Read the model definition and answer for the solid it produces. Units are mm, in the model's axes. Give positions to 0.01 mm unless a question says otherwise; leave off trailing zeros. Loops run counter-clockwise (first coordinate to the right, second up) from the corner with the lowest first, then second, coordinate; pieces in that order, holes last. Notation, with made-up numbers: (47, -30.75) -> (97, -30.75) arc R21 ccw to (97, 0.25) -> close; hole circle Ø1 at (-40, -27). An arc over 180 degrees is marked (long way). Return JSON: item names as keys, results as strings. Group by question number.
from build123d import *

# Parameters (mm, degrees)
SKETCH_1_R               = 35.5
EXTRUDE_1_DEPTH          = 3
CUT_EXTRUDE_1_REACH      = 193.4
SKETCH_3_R               = 2
PATTERN_CIRCULAR_1_COUNT = 10
MIRROR_1_COPY_1_REACH    = 193.4
MIRROR_1_COPY_1_SKETCH_R = 2
MIRROR_1_COPY_2_REACH    = 193.4
MIRROR_1_COPY_2_SKETCH_R = 2
MIRROR_1_COPY_3_REACH    = 193.4
MIRROR_1_COPY_3_SKETCH_R = 2
MIRROR_1_COPY_4_REACH    = 193.4
MIRROR_1_COPY_4_SKETCH_R = 2
MIRROR_1_COPY_5_REACH    = 193.4
MIRROR_1_COPY_5_SKETCH_R = 2
MIRROR_1_COPY_6_REACH    = 193.4
MIRROR_1_COPY_6_SKETCH_R = 2
MIRROR_1_COPY_7_REACH    = 193.4
MIRROR_1_COPY_7_SKETCH_R = 2
MIRROR_1_COPY_8_REACH    = 193.4
MIRROR_1_COPY_8_SKETCH_R = 2
MIRROR_1_COPY_9_REACH    = 193.4
MIRROR_1_COPY_9_SKETCH_R = 2
CUT_EXTRUDE_2_REACH      = 193.4
SKETCH_4_R               = 1.5
PATTERN_LINEAR_1_COUNT   = 5
PATTERN_LINEAR_1_PITCH   = 21
CUT_EXTRUDE_3_REACH      = 193.4
SKETCH_6_R               = 1.5
PATTERN_LINEAR_3_COUNT   = 5
PATTERN_LINEAR_3_PITCH   = 15
MIRROR_2_COPY_1_REACH    = 193.4
MIRROR_2_COPY_1_SKETCH_R = 1.5
MIRROR_2_COPY_2_REACH    = 193.4
MIRROR_2_COPY_2_SKETCH_R = 1.5
MIRROR_2_COPY_3_REACH    = 193.4
MIRROR_2_COPY_3_SKETCH_R = 1.5
MIRROR_2_COPY_4_REACH    = 193.4
MIRROR_2_COPY_4_SKETCH_R = 1.5
CUT_EXTRUDE_4_REACH      = 193.4
SKETCH_7_R               = 1.5
PATTERN_LINEAR_4_COUNT   = 2
PATTERN_LINEAR_4_PITCH   = 50


with BuildPart() as part:
    # Sketch 1 → Extrude 1 (new body)
    with BuildSketch(Plane(origin=(0, 0, 0), x_dir=(1, 0, 0), z_dir=(0, 1, 0))):
        with BuildLine():
            Line((-150, 65), (150, 65))
            ThreePointArc((150, 65), (171.213203436, 56.213203436), (180, 35))
            Line((180, 35), (180, -35))
            ThreePointArc((180, -35), (171.213203436, -56.213203436), (150, -65))
            Line((150, -65), (-150, -65))
            ThreePointArc((-150, -65), (-171.213203436, -56.213203436), (-180, -35))
            Line((-180, -35), (-180, 35))
            ThreePointArc((-180, 35), (-171.213203436, 56.213203436), (-150, 65))
        make_face()
        with Locations(Location((105, 0, 0), (0, 0, 270))):
            Circle(SKETCH_1_R, mode=Mode.SUBTRACT)
        with Locations(Location((-105, 0, 0), (0, 0, 270))):
            Circle(SKETCH_1_R, mode=Mode.SUBTRACT)
    extrude(amount=EXTRUDE_1_DEPTH)

    # Sketch 3 → Cut-Extrude 1 (cut, up to next)
    with BuildSketch(Plane(origin=(0, 3, 0), x_dir=(1, 0, 0), z_dir=(0, 1, 0)), mode=Mode.PRIVATE) as cut_extrude_1_sk1:
        with Locations(Location((-63, 0, 0), (0, 0, 270))):
            Circle(SKETCH_3_R)
    cut_extrude_1_tool1 = extrude(cut_extrude_1_sk1.sketch, amount=-CUT_EXTRUDE_1_REACH, mode=Mode.PRIVATE) & part.part
    cut_extrude_1 = cut_extrude_1_tool1.solids().sort_by_distance((-63, 3, 0))[0]
    add(cut_extrude_1, mode=Mode.SUBTRACT)

    # Pattern Circular 1: Cut-Extrude 1 ×10 about axis
    pattern_circular_1_axis = Axis((-105, 0, 0), (0, 1, 0))
    for i in range(1, PATTERN_CIRCULAR_1_COUNT):
        add(cut_extrude_1.rotate(pattern_circular_1_axis, i * 360 / PATTERN_CIRCULAR_1_COUNT), mode=Mode.SUBTRACT)

    # Mirror 1: Cut-Extrude 1 across plane
    add(cut_extrude_1.mirror(Plane(origin=(0, 0, 0), x_dir=(0, 0, 1), z_dir=(1, 0, 0))), mode=Mode.SUBTRACT)

    # Mirror 1 copy 1 sketch → Mirror 1 copy 1 (cut, up to next)
    with BuildSketch(Plane(origin=(20.053215591, 3, -61.717451491), x_dir=(-0.8090169943749475, 0, -0.5877852522924731), z_dir=(0, 1, 0)), mode=Mode.PRIVATE) as mirror_1_copy_1_sk1:
        with Locations((-63, 0)):
            Circle(MIRROR_1_COPY_1_SKETCH_R)
    mirror_1_copy_1_tool1 = extrude(mirror_1_copy_1_sk1.sketch, amount=-MIRROR_1_COPY_1_REACH, mode=Mode.PRIVATE) & part.part
    add(mirror_1_copy_1_tool1.solids().sort_by_distance((71.021286236, 3, -24.686980596))[0], mode=Mode.SUBTRACT)

    # Mirror 1 copy 2 sketch → Mirror 1 copy 2 (cut, up to next)
    with BuildSketch(Plane(origin=(72.553215591, 3, -99.860934211), x_dir=(-0.30901699437494745, 0, -0.9510565162951535), z_dir=(0, 1, 0)), mode=Mode.PRIVATE) as mirror_1_copy_2_sk1:
        with Locations((-63, 0)):
            Circle(MIRROR_1_COPY_2_SKETCH_R)
    mirror_1_copy_2_tool1 = extrude(mirror_1_copy_2_sk1.sketch, amount=-MIRROR_1_COPY_2_REACH, mode=Mode.PRIVATE) & part.part
    add(mirror_1_copy_2_tool1.solids().sort_by_distance((92.021286236, 3, -39.944373684))[0], mode=Mode.SUBTRACT)

    # Mirror 1 copy 3 sketch → Mirror 1 copy 3 (cut, up to next)
    with BuildSketch(Plane(origin=(137.446784409, 3, -99.860934211), x_dir=(0.30901699437494734, 0, -0.9510565162951536), z_dir=(0, 1, 0)), mode=Mode.PRIVATE) as mirror_1_copy_3_sk1:
        with Locations((-63, 0)):
            Circle(MIRROR_1_COPY_3_SKETCH_R)
    mirror_1_copy_3_tool1 = extrude(mirror_1_copy_3_sk1.sketch, amount=-MIRROR_1_COPY_3_REACH, mode=Mode.PRIVATE) & part.part
    add(mirror_1_copy_3_tool1.solids().sort_by_distance((117.978713764, 3, -39.944373684))[0], mode=Mode.SUBTRACT)

    # Mirror 1 copy 4 sketch → Mirror 1 copy 4 (cut, up to next)
    with BuildSketch(Plane(origin=(189.946784409, 3, -61.717451491), x_dir=(0.8090169943749473, 0, -0.5877852522924732), z_dir=(0, 1, 0)), mode=Mode.PRIVATE) as mirror_1_copy_4_sk1:
        with Locations((-63, 0)):
            Circle(MIRROR_1_COPY_4_SKETCH_R)
    mirror_1_copy_4_tool1 = extrude(mirror_1_copy_4_sk1.sketch, amount=-MIRROR_1_COPY_4_REACH, mode=Mode.PRIVATE) & part.part
    add(mirror_1_copy_4_tool1.solids().sort_by_distance((138.978713764, 3, -24.686980596))[0], mode=Mode.SUBTRACT)

    # Mirror 1 copy 5 sketch → Mirror 1 copy 5 (cut, up to next)
    with BuildSketch(Plane(origin=(210, 3, 0), x_dir=(1, 0, 0), z_dir=(0, 1, 0)), mode=Mode.PRIVATE) as mirror_1_copy_5_sk1:
        with Locations((-63, 0)):
            Circle(MIRROR_1_COPY_5_SKETCH_R)
    mirror_1_copy_5_tool1 = extrude(mirror_1_copy_5_sk1.sketch, amount=-MIRROR_1_COPY_5_REACH, mode=Mode.PRIVATE) & part.part
    add(mirror_1_copy_5_tool1.solids().sort_by_distance((147, 3, 0))[0], mode=Mode.SUBTRACT)

    # Mirror 1 copy 6 sketch → Mirror 1 copy 6 (cut, up to next)
    with BuildSketch(Plane(origin=(189.946784409, 3, 61.717451491), x_dir=(0.8090169943749476, 0, 0.587785252292473), z_dir=(0, 1, 0)), mode=Mode.PRIVATE) as mirror_1_copy_6_sk1:
        with Locations((-63, 0)):
            Circle(MIRROR_1_COPY_6_SKETCH_R)
    mirror_1_copy_6_tool1 = extrude(mirror_1_copy_6_sk1.sketch, amount=-MIRROR_1_COPY_6_REACH, mode=Mode.PRIVATE) & part.part
    add(mirror_1_copy_6_tool1.solids().sort_by_distance((138.978713764, 3, 24.686980596))[0], mode=Mode.SUBTRACT)

    # Mirror 1 copy 7 sketch → Mirror 1 copy 7 (cut, up to next)
    with BuildSketch(Plane(origin=(137.446784409, 3, 99.860934211), x_dir=(0.30901699437494756, 0, 0.9510565162951535), z_dir=(0, 1, 0)), mode=Mode.PRIVATE) as mirror_1_copy_7_sk1:
        with Locations((-63, 0)):
            Circle(MIRROR_1_COPY_7_SKETCH_R)
    mirror_1_copy_7_tool1 = extrude(mirror_1_copy_7_sk1.sketch, amount=-MIRROR_1_COPY_7_REACH, mode=Mode.PRIVATE) & part.part
    add(mirror_1_copy_7_tool1.solids().sort_by_distance((117.978713764, 3, 39.944373684))[0], mode=Mode.SUBTRACT)

    # Mirror 1 copy 8 sketch → Mirror 1 copy 8 (cut, up to next)
    with BuildSketch(Plane(origin=(72.553215591, 3, 99.860934211), x_dir=(-0.30901699437494723, 0, 0.9510565162951536), z_dir=(0, 1, 0)), mode=Mode.PRIVATE) as mirror_1_copy_8_sk1:
        with Locations((-63, 0)):
            Circle(MIRROR_1_COPY_8_SKETCH_R)
    mirror_1_copy_8_tool1 = extrude(mirror_1_copy_8_sk1.sketch, amount=-MIRROR_1_COPY_8_REACH, mode=Mode.PRIVATE) & part.part
    add(mirror_1_copy_8_tool1.solids().sort_by_distance((92.021286236, 3, 39.944373684))[0], mode=Mode.SUBTRACT)

    # Mirror 1 copy 9 sketch → Mirror 1 copy 9 (cut, up to next)
    with BuildSketch(Plane(origin=(20.053215591, 3, 61.717451491), x_dir=(-0.8090169943749473, 0, 0.5877852522924734), z_dir=(0, 1, 0)), mode=Mode.PRIVATE) as mirror_1_copy_9_sk1:
        with Locations((-63, 0)):
            Circle(MIRROR_1_COPY_9_SKETCH_R)
    mirror_1_copy_9_tool1 = extrude(mirror_1_copy_9_sk1.sketch, amount=-MIRROR_1_COPY_9_REACH, mode=Mode.PRIVATE) & part.part
    add(mirror_1_copy_9_tool1.solids().sort_by_distance((71.021286236, 3, 24.686980596))[0], mode=Mode.SUBTRACT)

    # Sketch 4 → Cut-Extrude 2 (cut, up to next)
    with BuildSketch(Plane(origin=(0, 3, 0), x_dir=(1, 0, 0), z_dir=(0, 1, 0)), mode=Mode.PRIVATE) as cut_extrude_2_sk1:
        with Locations(Location((42, 50, 0), (0, 0, 270))):
            Circle(SKETCH_4_R)
    cut_extrude_2_tool1 = extrude(cut_extrude_2_sk1.sketch, amount=-CUT_EXTRUDE_2_REACH, mode=Mode.PRIVATE) & part.part
    cut_extrude_2 = cut_extrude_2_tool1.solids().sort_by_distance((42, 3, -50))[0]
    add(cut_extrude_2, mode=Mode.SUBTRACT)

    # Pattern Linear 1: Cut-Extrude 2 ×5
    with Locations(*[(-i * PATTERN_LINEAR_1_PITCH, 0, 0) for i in range(1, PATTERN_LINEAR_1_COUNT)]):
        add(cut_extrude_2, mode=Mode.SUBTRACT)

    # Sketch 6 → Cut-Extrude 3 (cut, up to next)
    with BuildSketch(Plane(origin=(0, 3, 0), x_dir=(1, 0, 0), z_dir=(0, 1, 0)), mode=Mode.PRIVATE) as cut_extrude_3_sk1:
        with Locations(Location((30, 29.5, 0), (0, 0, 270))):
            Circle(SKETCH_6_R)
    cut_extrude_3_tool1 = extrude(cut_extrude_3_sk1.sketch, amount=-CUT_EXTRUDE_3_REACH, mode=Mode.PRIVATE) & part.part
    cut_extrude_3 = cut_extrude_3_tool1.solids().sort_by_distance((30, 3, -29.5))[0]
    add(cut_extrude_3, mode=Mode.SUBTRACT)

    # Pattern Linear 3: Cut-Extrude 3 ×5
    with Locations(*[(-i * PATTERN_LINEAR_3_PITCH, 0, 0) for i in range(1, PATTERN_LINEAR_3_COUNT)]):
        add(cut_extrude_3, mode=Mode.SUBTRACT)

    # Mirror 2: Cut-Extrude 3 across plane
    add(cut_extrude_3.mirror(Plane.XY), mode=Mode.SUBTRACT)

    # Mirror 2 copy 1 sketch → Mirror 2 copy 1 (cut, up to next)
    with BuildSketch(Plane(origin=(-15, 3, 0), x_dir=(1, 0, 0), z_dir=(0, 1, 0)), mode=Mode.PRIVATE) as mirror_2_copy_1_sk1:
        with Locations((30, -29.5)):
            Circle(MIRROR_2_COPY_1_SKETCH_R)
    mirror_2_copy_1_tool1 = extrude(mirror_2_copy_1_sk1.sketch, amount=-MIRROR_2_COPY_1_REACH, mode=Mode.PRIVATE) & part.part
    add(mirror_2_copy_1_tool1.solids().sort_by_distance((15, 3, 29.5))[0], mode=Mode.SUBTRACT)

    # Mirror 2 copy 2 sketch → Mirror 2 copy 2 (cut, up to next)
    with BuildSketch(Plane(origin=(-30, 3, 0), x_dir=(1, 0, 0), z_dir=(0, 1, 0)), mode=Mode.PRIVATE) as mirror_2_copy_2_sk1:
        with Locations((30, -29.5)):
            Circle(MIRROR_2_COPY_2_SKETCH_R)
    mirror_2_copy_2_tool1 = extrude(mirror_2_copy_2_sk1.sketch, amount=-MIRROR_2_COPY_2_REACH, mode=Mode.PRIVATE) & part.part
    add(mirror_2_copy_2_tool1.solids().sort_by_distance((0, 3, 29.5))[0], mode=Mode.SUBTRACT)

    # Mirror 2 copy 3 sketch → Mirror 2 copy 3 (cut, up to next)
    with BuildSketch(Plane(origin=(-45, 3, 0), x_dir=(1, 0, 0), z_dir=(0, 1, 0)), mode=Mode.PRIVATE) as mirror_2_copy_3_sk1:
        with Locations((30, -29.5)):
            Circle(MIRROR_2_COPY_3_SKETCH_R)
    mirror_2_copy_3_tool1 = extrude(mirror_2_copy_3_sk1.sketch, amount=-MIRROR_2_COPY_3_REACH, mode=Mode.PRIVATE) & part.part
    add(mirror_2_copy_3_tool1.solids().sort_by_distance((-15, 3, 29.5))[0], mode=Mode.SUBTRACT)

    # Mirror 2 copy 4 sketch → Mirror 2 copy 4 (cut, up to next)
    with BuildSketch(Plane(origin=(-60, 3, 0), x_dir=(1, 0, 0), z_dir=(0, 1, 0)), mode=Mode.PRIVATE) as mirror_2_copy_4_sk1:
        with Locations((30, -29.5)):
            Circle(MIRROR_2_COPY_4_SKETCH_R)
    mirror_2_copy_4_tool1 = extrude(mirror_2_copy_4_sk1.sketch, amount=-MIRROR_2_COPY_4_REACH, mode=Mode.PRIVATE) & part.part
    add(mirror_2_copy_4_tool1.solids().sort_by_distance((-30, 3, 29.5))[0], mode=Mode.SUBTRACT)

    # Sketch 7 → Cut-Extrude 4 (cut, up to next)
    with BuildSketch(Plane(origin=(0, 3, 0), x_dir=(1, 0, 0), z_dir=(0, 1, 0)), mode=Mode.PRIVATE) as cut_extrude_4_sk1:
        with Locations(Location((42, 0, 0), (0, 0, 270))):
            Circle(SKETCH_7_R)
    cut_extrude_4_tool1 = extrude(cut_extrude_4_sk1.sketch, amount=-CUT_EXTRUDE_4_REACH, mode=Mode.PRIVATE) & part.part
    # Sketch 7 → Cut-Extrude 4 (cut, up to next)
    with BuildSketch(Plane(origin=(0, 3, 0), x_dir=(1, 0, 0), z_dir=(0, 1, 0)), mode=Mode.PRIVATE) as cut_extrude_4_sk2:
        with Locations(Location((0, 0, 0), (0, 0, 270))):
            Circle(SKETCH_7_R)
    cut_extrude_4_tool2 = extrude(cut_extrude_4_sk2.sketch, amount=-CUT_EXTRUDE_4_REACH, mode=Mode.PRIVATE) & part.part
    # Sketch 7 → Cut-Extrude 4 (cut, up to next)
    with BuildSketch(Plane(origin=(0, 3, 0), x_dir=(1, 0, 0), z_dir=(0, 1, 0)), mode=Mode.PRIVATE) as cut_extrude_4_sk3:
        with Locations(Location((-42, 0, 0), (0, 0, 270))):
            Circle(SKETCH_7_R)
    cut_extrude_4_tool3 = extrude(cut_extrude_4_sk3.sketch, amount=-CUT_EXTRUDE_4_REACH, mode=Mode.PRIVATE) & part.part
    cut_extrude_4_1 = cut_extrude_4_tool1.solids().sort_by_distance((42, 3, 0))[0]
    add(cut_extrude_4_1, mode=Mode.SUBTRACT)
    cut_extrude_4_2 = cut_extrude_4_tool2.solids().sort_by_distance((0, 3, 0))[0]
    add(cut_extrude_4_2, mode=Mode.SUBTRACT)
    cut_extrude_4_3 = cut_extrude_4_tool3.solids().sort_by_distance((-42, 3, 0))[0]
    add(cut_extrude_4_3, mode=Mode.SUBTRACT)
    cut_extrude_4 = cut_extrude_4_1 + cut_extrude_4_2 + cut_extrude_4_3  # Cut-Extrude 4 as one shape, for the pattern or mirror that repeats it

    # Pattern Linear 4: Cut-Extrude 4 ×2
    with Locations(*[(0, 0, i * PATTERN_LINEAR_4_PITCH) for i in range(1, PATTERN_LINEAR_4_COUNT)]):
        add(cut_extrude_4, mode=Mode.SUBTRACT)


solid = part.part
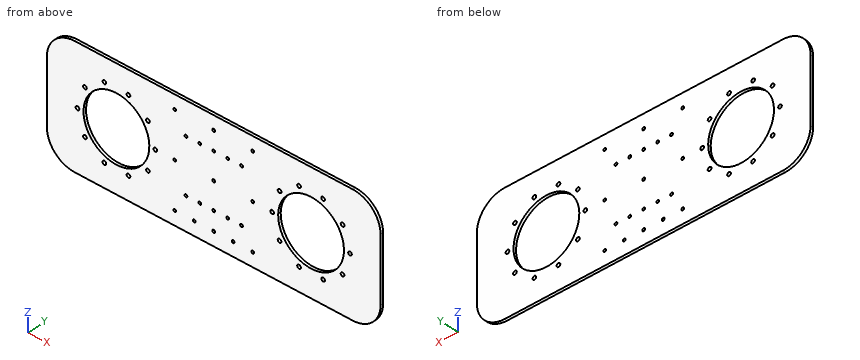
1. Section A-A on x = 105 is taken. Determine the outline of the cut face in (y, z).
2. Section D-D on z = 7 is taken. Determine the outline of the cut face in (x, y).
3. Straight lines are drawn through the part: line 1 (X direction, y = 2.55, z = 15.5); line 2 (X direction, y = 1.35, z = 22.5); line 3 (Z direction, x = -15.5, y = 0.1). For each, find the intervals that lie inside material, in ascending order. Write a range as from..to.
4. A flat-ended cylindrical pin translates along its axis: pin 1 Ø2.5 at (x, z) = (30, 29.5) entering from +Y. Find the tip coordinate at first contact, or state that the pin passes through.
5. Section B-B on z = -9 is taken. Determine the outline of the cut face in (x, y).
6. Section C-C on y = 2.3 is taken. State how many separate pieces and enclosed holes the cut face has, then the cut area to 3 significant figures.
Completed:
{
 "1": {"outline": "(0, -65) -> (3, -65) -> (3, -35.5) -> (0, -35.5) -> close; (0, 35.5) -> (3, 35.5) -> (3, 65) -> (0, 65) -> close"},
 "2": {"outline": "(-180, 0) -> (-139.8, 0) -> (-139.8, 3) -> (-180, 3) -> close; (-70.2, 0) -> (70.2, 0) -> (70.2, 3) -> (-70.2, 3) -> close; (139.8, 0) -> (180, 0) -> (180, 3) -> (139.8, 3) -> close"},
 "3": {"line 1": "x = -180..-136.94, -73.06..73.06, 136.94..180", "line 2": "x = -180..-132.46, -77.54..77.54, 132.46..180", "line 3": "z = -65..-30.91, -28.09..28.09, 30.91..65"},
 "4": {"pin 1": "passes through"},
 "5": {"outline": "(-180, 0) -> (-139.34, 0) -> (-139.34, 3) -> (-180, 3) -> close; (-70.66, 0) -> (70.66, 0) -> (70.66, 3) -> (-70.66, 3) -> close; (139.34, 0) -> (180, 0) -> (180, 3) -> (139.34, 3) -> close"},
 "6": {"separate pieces": "1", "enclosed holes": "43", "area": "37,700 mm²"}
}
